CAD build for the part. Positions are in the model's coordinates, mm. Face numbers are marked on the shaded views. A direction names the side the tool comes from. Give positions to 0.01 mm unless a question says otherwise; leave off trailing zeros. Loops run counter-clockwise (first coordinate to the right, second up) from the corner with the lowest first, then second, coordinate; pieces in that order, holes last.
```python
from build123d import *

# Parameters (mm, degrees)
F0_W     = 270
F0_H     = 200
F1_DEPTH = 355
F2_T     = -1.5


with BuildPart() as f1:
    # F0 (on Right) → F1 (new body)
    with BuildSketch(Plane.YZ):
        with Locations((135, 100)):
            Rectangle(F0_W, F0_H)
    extrude(amount=-F1_DEPTH)

    # F2
    f2_openings = [f1.faces().sort_by_distance(p)[0] for p in [
        (-177.5, 0, 100),
    ]]
    offset(amount=F2_T, openings=f2_openings)


solid = f1.part
```
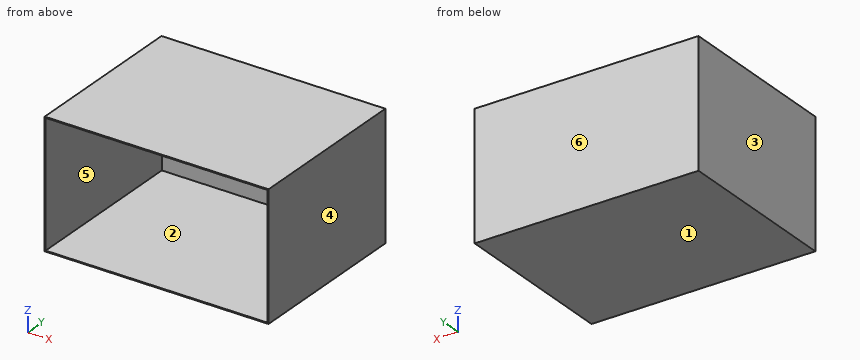
1. Saw through at B-B, the plane z = 171. List the corners of the cut face in (x, y), and give its area (3 significant figures).
Responses:
outline: (-355, 0) - (-353.5, 0) - (-353.5, 268.5) - (-1.5, 268.5) - (-1.5, 0) - (0, 0) - (0, 270) - (-355, 270) - close
area: 1,340 mm2
2. Saw through at C-C, the plane x = -332.5. List the corners of the cut face in (y, z), and give its area (3 significant figures).
Responses:
outline: (0, 0) - (270, 0) - (270, 200) - (0, 200) - (0, 198.5) - (268.5, 198.5) - (268.5, 1.5) - (0, 1.5) - close
area: 1,110 mm2
3. Drop flat-ended pins along their axis: pin 1 (6 mm diameter, centred on y = 216, z = 114, fed in from +X); pin 2 (4 mm diameter, centred on x = -136, z = 168, fed in from -Y). Give the stop position or say it passes through.
Responses:
pin 1: stops at x = 0
pin 2: stops at y = 268.5
4. Saw through at A-A, the plane y = 134.5. List the corners of the cut face in (x, z), and give its area (3 significant figures).
Responses:
outline: (-355, 0) - (0, 0) - (0, 200) - (-355, 200) - close; hole (-353.5, 1.5) - (-1.5, 1.5) - (-1.5, 198.5) - (-353.5, 198.5) - close
area: 1,660 mm2
5. Tool access for the marked faces 5 and 6: list every direction of +Z, -Z, +X, -X, +Y, -Y with a clear straight run to the whole face (end or side of a thin tool).
Responses:
face 5: -Y
face 6: +Z, -Z, +X, -X, +Y
6. Pull direction X, two halves, no side cores. Call the marked faces 1, 2, 3 and 4: released by +X, released by -X, zero draft, split by the parting line, or undercut.
Responses:
face 1: zero draft
face 2: undercut
face 3: released by -X
face 4: released by +X
7. Probe line 1 along Z through (x, y) = (-76.5, 122); line 2 along X through (y, z) = (187, 166); line 3 along Y through (x, z) = (-158.5, 71.5). List the from-to ranges inside material, lowest first.
Responses:
line 1: z = 0 to 1.5, 198.5 to 200
line 2: x = -355 to -353.5, -1.5 to 0
line 3: y = 268.5 to 270
